For this review, take the finished solid that the model builds, in its own axes (mm). A direction names the side the tool comes from. Give positions to 0.01 mm unless a question says otherwise; leave off trailing zeros. Write each loop counter-clockwise with the first axis right and the second up, starting at its lowest first coordinate (ties: lowest second). Pieces come first, ordered by that corner, then holes.
1) We need section B-B on x = -1.5. Give the boundary of the cut face in (y, z).
2) Draft analysis for pull direction Z (two halves, no side actions). For faces 5 (the face through (33.55, 83.67, -7.7)), 6 (the face through (-2, 50, 43.251)), 7 (the face through (-36, 0, 5)), state which applies: pulls with the +Z half, pulls with the -Z half, needs draft (parallel to the pull), parting line crosses it, or undercut.
3) We need section A-A on y = 29. Give the boundary of the cut face in (x, z), and give its area (3 significant figures).
4) Wall thickness on line 1 along Z through (x, y) = (19, 66); line 2 along X through (y, z) = (14, -15.5); line 3 along Z through (x, y) = (32, 32.5): over which ranges is each line inside the solid? List them lowest first.
5) We need section C-C on z = -21. Give the boundary of the cut face in (x, y).
6) We need section D-D on y = 63. Give the boundary of the cut face in (x, z), and give its area (3 significant figures).
7) For P1, Ø2, axis at y = 3.18, z = 11.5, coming from the -X side; P2, Ø1.4, axis at y = 82.55, z = 17.85, coming from the +X side, all flat-tipped, find the tip position at first contact; note any pin that passes through.
8) Machinability: for faces 1 (the face through (-24.948, 22.226, 40.12)), 2 (the face through (-33.082, 52, 6)), 3 (the face through (-36.3, 3.22, 10.37)), 4 (the face through (33.637, 53.974, -13.207)), which of the approach directions +Z, -Z, +X, -X, +Y, -Y give a long, thin tool a straight path to every point of the face, cutting with its end or side? Answer none if there is none.
from build123d import *

# Parameters (mm, degrees)
SKETCH2_W                 = 76.2
SKETCH2_H                 = 76.2
BOSS_EXTRUDE1_DEPTH       = 101.6
SKETCH3_W                 = 63.5
SKETCH3_H                 = 63.5
CUT_EXTRUDE1_DEPTH        = 102.6
CUT_EXTRUDE2_REACH        = 78.2
CUT_EXTRUDE3_REACH        = 78.2
F_4_40_TAPPED_HOLE1_D     = 2.2606
F_4_40_TAPPED_HOLE1_DEPTH = 6.35
F_4_40_TAPPED_HOLE2_D     = 2.2606
F_4_40_TAPPED_HOLE2_DEPTH = 6.35
F_4_40_TAPPED_HOLE3_D     = 2.2606


with BuildPart() as part:
    # Sketch2 → Boss-Extrude1 (new body)
    with BuildSketch(Plane(origin=(0, 0, 0), x_dir=(1, 0, 0), z_dir=(0, 1, 0))):
        with Locations((-1.332167832, -5.151048951)):
            Rectangle(SKETCH2_W, SKETCH2_H)
    extrude(amount=BOSS_EXTRUDE1_DEPTH)

    # Sketch3 → Cut-Extrude1 (cut, through all)
    with BuildSketch(Plane(origin=(0, 101.6, 0), x_dir=(1, 0, 0), z_dir=(0, 1, 0))):
        with Locations((-1.332167832, -5.151048951)):
            Rectangle(SKETCH3_W, SKETCH3_H)
    extrude(amount=-CUT_EXTRUDE1_DEPTH, mode=Mode.SUBTRACT)

    # Sketch4 → Cut-Extrude2 (cut, up to next)
    with BuildSketch(Plane.XY.offset(43.251048951), mode=Mode.PRIVATE) as cut_extrude2_sk1:
        with BuildLine():
            Line((-28.192667832, 25.4), (-28.192667832, 50.8))
            ThreePointArc((-28.192667832, 50.8), (-25.017667832, 53.975), (-21.842667832, 50.8))
            Line((-21.842667832, 50.8), (-21.842667832, 25.4))
            ThreePointArc((-21.842667832, 25.4), (-25.017667832, 22.225), (-28.192667832, 25.4))
        make_face()
    cut_extrude2_tool1 = extrude(cut_extrude2_sk1.sketch, amount=-CUT_EXTRUDE2_REACH, mode=Mode.PRIVATE) & part.part
    add(cut_extrude2_tool1.solids().sort_by_distance((-25.017668, 38.1, 43.251049))[0], mode=Mode.SUBTRACT)
    # Sketch4 → Cut-Extrude2 (cut, up to next)
    with BuildSketch(Plane.XY.offset(43.251048951), mode=Mode.PRIVATE) as cut_extrude2_sk2:
        with BuildLine():
            Line((20.829332168, 25.4), (20.829332168, 50.8))
            ThreePointArc((20.829332168, 50.8), (24.004332168, 53.975), (27.179332168, 50.8))
            Line((27.179332168, 50.8), (27.179332168, 25.4))
            ThreePointArc((27.179332168, 25.4), (24.004332168, 22.225), (20.829332168, 25.4))
        make_face()
    cut_extrude2_tool2 = extrude(cut_extrude2_sk2.sketch, amount=-CUT_EXTRUDE2_REACH, mode=Mode.PRIVATE) & part.part
    add(cut_extrude2_tool2.solids().sort_by_distance((24.004332, 38.1, 43.251049))[0], mode=Mode.SUBTRACT)

    # Sketch5 → Cut-Extrude3 (cut, up to next)
    with BuildSketch(Plane(origin=(36.767832168, 0, 0), x_dir=(0, 0, -1), z_dir=(1, 0, 0)), mode=Mode.PRIVATE) as cut_extrude3_sk1:
        with BuildLine():
            Line((-32.824348951, 25.4), (-32.824348951, 50.8))
            ThreePointArc((-32.824348951, 50.8), (-29.649348951, 53.975), (-26.474348951, 50.8))
            Line((-26.474348951, 50.8), (-26.474348951, 25.4))
            ThreePointArc((-26.474348951, 25.4), (-29.649348951, 22.225), (-32.824348951, 25.4))
        make_face()
    cut_extrude3_tool1 = extrude(cut_extrude3_sk1.sketch, amount=-CUT_EXTRUDE3_REACH, mode=Mode.PRIVATE) & part.part
    add(cut_extrude3_tool1.solids().sort_by_distance((36.767832, 38.1, 29.649349))[0], mode=Mode.SUBTRACT)
    # Sketch5 → Cut-Extrude3 (cut, up to next)
    with BuildSketch(Plane(origin=(36.767832168, 0, 0), x_dir=(0, 0, -1), z_dir=(1, 0, 0)), mode=Mode.PRIVATE) as cut_extrude3_sk2:
        with BuildLine():
            Line((10.101651049, 25.4), (10.101651049, 50.8))
            ThreePointArc((10.101651049, 50.8), (13.276651049, 53.975), (16.451651049, 50.8))
            Line((16.451651049, 50.8), (16.451651049, 25.4))
            ThreePointArc((16.451651049, 25.4), (13.276651049, 22.225), (10.101651049, 25.4))
        make_face()
    cut_extrude3_tool2 = extrude(cut_extrude3_sk2.sketch, amount=-CUT_EXTRUDE3_REACH, mode=Mode.PRIVATE) & part.part
    add(cut_extrude3_tool2.solids().sort_by_distance((36.767832, 38.1, -13.276651))[0], mode=Mode.SUBTRACT)

    # #4-40 Tapped Hole1
    with Locations(Plane.XY.offset(43.251048951)):
        with Locations((-14.032167832, 82.55), (11.367832168, 82.55)):
            Hole(F_4_40_TAPPED_HOLE1_D / 2, depth=F_4_40_TAPPED_HOLE1_DEPTH)

    # #4-40 Tapped Hole2
    with Locations(Plane(origin=(36.767832168, 0, 0), x_dir=(0, 0, -1), z_dir=(1, 0, 0))):
        with Locations((-17.851048951, 82.55), (7.548951049, 82.55)):
            Hole(F_4_40_TAPPED_HOLE2_D / 2, depth=F_4_40_TAPPED_HOLE2_DEPTH)

    # #4-40 Tapped Hole3 (through all)
    with Locations(Plane(origin=(36.767832168, 0, 0), x_dir=(0, 0, -1), z_dir=(1, 0, 0))):
        with Locations((1.198951049, 3.175), (-11.501048951, 3.175)):
            Hole(F_4_40_TAPPED_HOLE3_D / 2)


solid = part.part
Results list:
1. outline: (0, -32.95) - (101.6, -32.95) - (101.6, -26.6) - (0, -26.6) - close; (0, 36.9) - (101.6, 36.9) - (101.6, 43.25) - (0, 43.25) - close
2. face 5: undercut
2. face 6: pulls with the +Z half
2. face 7: needs draft
3. outline: (-39.43, -32.95) - (36.77, -32.95) - (36.77, -16.45) - (30.42, -16.45) - (30.42, -26.6) - (-33.08, -26.6) - (-33.08, 36.9) - (-28.19, 36.9) - (-28.19, 43.25) - (-39.43, 43.25) - close; (-21.84, 36.9) - (20.83, 36.9) - (20.83, 43.25) - (-21.84, 43.25) - close; (27.18, 36.9) - (30.42, 36.9) - (30.42, 32.82) - (36.77, 32.82) - (36.77, 43.25) - (27.18, 43.25) - close; (30.42, -10.1) - (36.77, -10.1) - (36.77, 26.47) - (30.42, 26.47) - close
3. area: 1,610 mm2
4. line 1: z = -32.95 to -26.6, 36.9 to 43.25
4. line 2: x = -39.43 to -33.08, 30.42 to 36.77
4. line 3: z = -32.95 to -16.45, -10.1 to 26.47, 32.82 to 43.25
5. outline: (-39.43, 0) - (-33.08, 0) - (-33.08, 101.6) - (-39.43, 101.6) - close; (30.42, 0) - (36.77, 0) - (36.77, 101.6) - (30.42, 101.6) - close
6. outline: (-39.43, -32.95) - (36.77, -32.95) - (36.77, 43.25) - (-39.43, 43.25) - close; hole (-33.08, -26.6) - (30.42, -26.6) - (30.42, 36.9) - (-33.08, 36.9) - close
6. area: 1,770 mm2
7. P1: passes through
7. P2: stops at x = -33.08
8. face 1: +Z
8. face 2: +Y, -Y
8. face 3: +X, -X
8. face 4: +X
